CAD build for the part. Positions are in the model's coordinates, mm. Face numbers are marked on the shaded views. Round coordinates to 2 decimals unless told otherwise and drop trailing zeros. Loops run counter-clockwise (first coordinate to the right, second up) from the corner with the lowest first, then second, coordinate; pieces in that order, holes last.
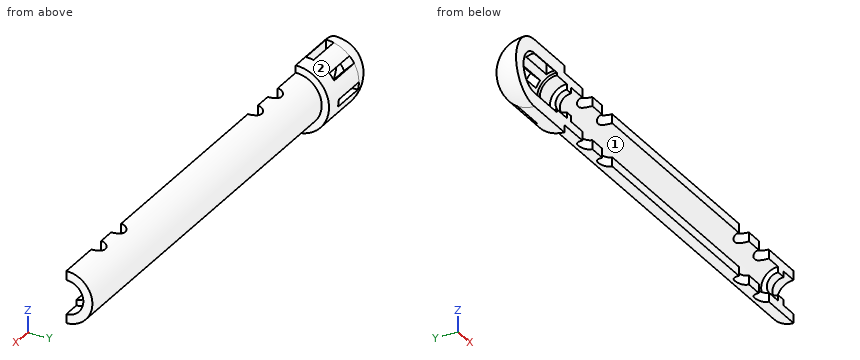
from build123d import *

# Parameters (mm, degrees)
REVOLVE6_ANGLE          = 180
SKETCH2_W               = 8.091492299
SKETCH2_H               = 1.703338147
CUT_EXTRUDE1_DEPTH      = 10
CIRPATTERN1_COUNT       = 8
CUT_EXTRUDE4_DEPTH      = 80.570407996
CUT_EXTRUDE4_DEPTH_BACK = 80.570407996
SKETCH3_R               = 2


with BuildPart() as part:
    # Sketch1 → Revolve6 (revolve)
    with BuildSketch(Plane(origin=(0, 0, 0), x_dir=(1, 0, 0), z_dir=(0, 1, 0))):
        with BuildLine():
            Line((-7.909078058, 1.25), (72.378975497, 1.25))
            Line((72.378975497, 1.25), (72.378975497, 0))
            Line((72.378975497, 0), (74.608975497, 0))
            Line((74.608975497, 0), (74.608975497, 1.25))
            Line((74.608975497, 1.25), (78.608975497, 1.25))
            Line((78.608975497, 1.25), (78.608975497, 3.25))
            Line((78.608975497, 3.25), (74.913959146, 3.25))
            Line((74.913959146, 3.25), (-13.655190787, 3.25))
            Line((-13.655190787, 3.25), (-13.655190787, 4.88))
            Line((-13.655190787, 4.88), (-16.655190787, 4.88))
            Line((-16.655190787, 4.88), (-25.666337235, 4.88))
            ThreePointArc((-25.666337235, 4.88), (-30.88478528, 2.718448045), (-33.046337235, -2.5))
            Line((-33.046337235, -2.5), (-30.045517155, -2.5))
            ThreePointArc((-30.045517155, -2.5), (-28.762885052, 0.596547817), (-25.666337235, 1.87917992))
            Line((-25.666337235, 1.87917992), (-16.655190787, 1.87917992))
            Line((-16.655190787, 1.87917992), (-16.655190787, 1.25))
            Line((-16.655190787, 1.25), (-12.635190787, 1.25))
            Line((-12.635190787, 1.25), (-12.635190787, 0))
            Line((-12.635190787, 0), (-10.905190787, 0))
            Line((-10.905190787, 0), (-10.905190787, 1.25))
            Line((-10.905190787, 1.25), (-7.909078058, 1.25))
        make_face()
    revolve(axis=Axis((-33.046337235, 0, 2.5), (1, 0, 0)), revolution_arc=REVOLVE6_ANGLE)

    # Sketch2 → Cut-Extrude1 (cut)
    with BuildSketch(Plane(origin=(0, 0, 0), x_dir=(1, 0, 0), z_dir=(0, 1, 0))):
        with Locations((-21.620591086, -1.552211442)):
            Rectangle(SKETCH2_W, SKETCH2_H)
    cut_extrude1 = extrude(amount=CUT_EXTRUDE1_DEPTH, mode=Mode.SUBTRACT)

    # CirPattern1: Cut-Extrude1 ×8 about axis
    cirpattern1_axis = Axis((0, 0, 2.5), (1, 0, 0))
    for i in range(1, CIRPATTERN1_COUNT):
        add(cut_extrude1.rotate(cirpattern1_axis, i * 360 / CIRPATTERN1_COUNT), mode=Mode.SUBTRACT)

    # Sketch3 → Cut-Extrude4 (cut, two sides: drawn at the far end of the back side and taken through both)
    with BuildSketch(Plane.XY.offset(-CUT_EXTRUDE4_DEPTH_BACK)):
        with Locations((66.608975497, 0)):
            Circle(SKETCH3_R)
        with Locations((58.608975497, 0)):
            Circle(SKETCH3_R)
        with Locations((3.608975497, 0)):
            Circle(SKETCH3_R)
        with Locations((-4.391024503, 0)):
            Circle(SKETCH3_R)
    extrude(amount=CUT_EXTRUDE4_DEPTH + CUT_EXTRUDE4_DEPTH_BACK, mode=Mode.SUBTRACT)


solid = part.part
Item 1: Flat gauge pins, fed straight in: P1, Ø1, axis at x = 49.5, z = 7, coming from the +Y side; P2, Ø0.9, axis at x = -23, y = 5.5, coming from the -Z side; P3, Ø1.6, axis at y = 4, z = 6.5, coming from the -X side. Where does each tip first touch, or does it go through?
Verdict:
P1: stops at y = 4.13
P2: stops at z = -2.79
P3: stops at x = -31.22
Item 2: Mould opens along Z. For the marked faces 1 and 2 say: released by +Z, released by -Z, zero draft, split by the parting line, or undercut.
Verdict:
face 1: undercut
face 2: split by the parting line
Item 3: Wall check: L1, parallel to X at y = 2.25, z = 0; L2, parallel to Y at x = -1, z = 2.75; L3, parallel to Z at x = 35.5, y = 1. Give the ranges that are in metal, low to high.
Verdict:
L1: x = -32.24 to -28.47, -12.64 to -10.91, 72.38 to 74.61
L2: y = 3.74 to 5.74
L3: z = -3.16 to -1.11, 6.11 to 8.16
Item 4: Cut at A-A (x = 54). List the corners of the cut face in (y, z), plus the area to 3 significant figures.
Verdict:
outline: (0, -3.25) arc R5.75 ccw to (0, 8.25) - (0, 6.25) arc R3.75 cw to (0, -1.25) - close
area: 29.8 mm2
